Geometry: see drawing. Coordinates: mm, zero at the bounding-box minimum. A direction names the side the tool comes from. Give positions to 0.01 mm unless a question says otherwise; leave off trailing zeros. Write each loop counter-clockwise with the first axis right and the second up, starting at its lowest first coordinate (ties: lowest second). Pieces come first, ordered by that corner, then holes.
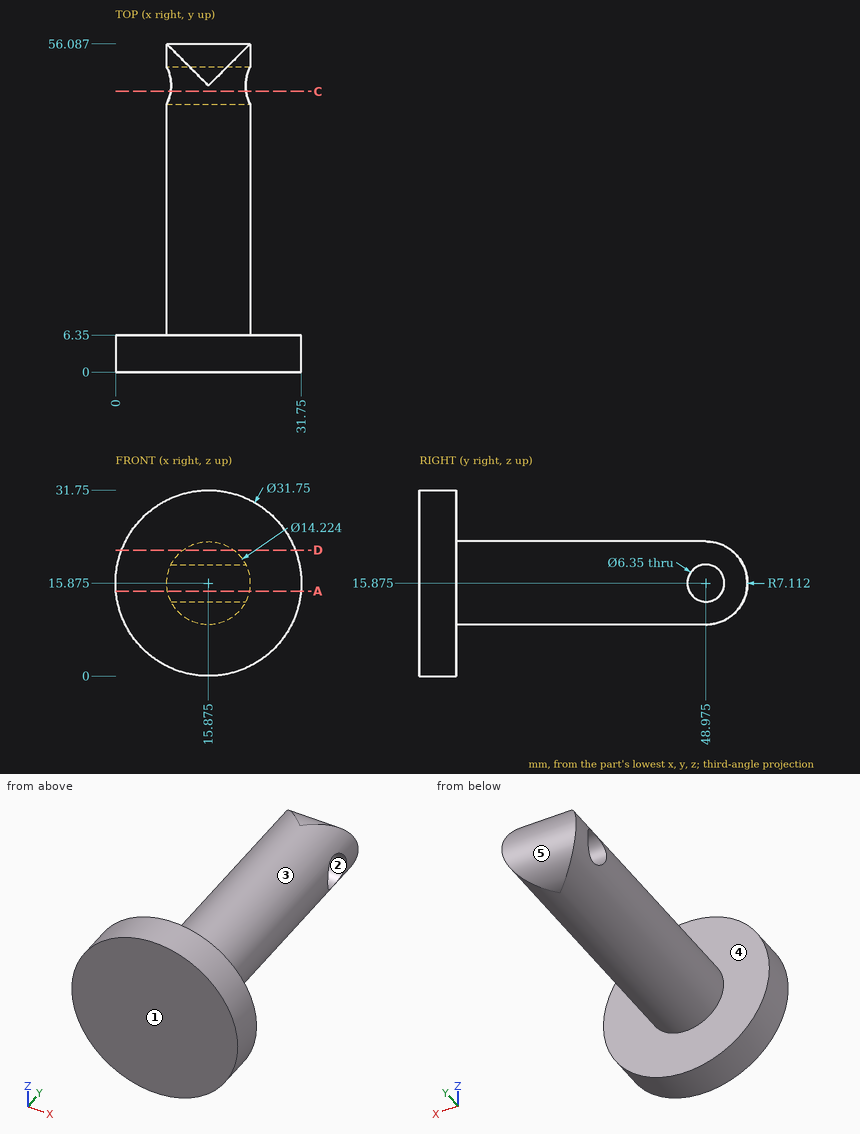
Q1. Access query for the marked faces 4 and 5. Directions: +Z, -Z, +X, -X, +Y, -Y. A direction counts if a zero-diameter tool reaches every point of the face in a straight line with its end or side. Return the directions, or none.
Q2. Section D-D, the plane z = 21.5. Return the cut outline in (x, y), then the cut area to 3 significant figures.
Q3. Material intervals for line 1 along Y through (x, z) = (22.5, 16); line 2 along Y through (x, z) = (9, 9); line 3 along Z through (x, y) = (12, 48), sorted ascending.
Q4. Section C-C, the plane y = 48. Return the cut outline in (x, z) (1 decimal).
Q5. Pin query (flat end, axial travel): pin 1 (6 mm diameter, centred on x = 22, z = 10.5, fed in from +Y); pin 2 (12 mm diameter, centred on x = 10.5, y = 40.5, fed in from +Z); pin 3 (2 mm diameter, centred on x = 22, z = 10, fed in from +Y); pin 4 (4 mm diameter, centred on y = 48.97, z = 15.88, fed in from +X). Return the tip coordinate at first contact, or that it passes through.
Q6. Mould query, pull axis Z, two halves, no side actions, for the marked faces 1, 2 and 3. Classes: +Z half, -Z half, draft (parallel to the pull), parting line (faces both ways), or undercut.
Q7. Section A-A, the plane z = 14.5. Return the cut outline in (x, y), then the cut area to 3 significant figures.
Solutions:
1. face 4: +Y
1. face 5: +X, -X, +Y
2. outline: (1.03, 0) - (30.72, 0) - (30.72, 6.35) - (20.23, 6.35) - (20.23, 53.33) - (11.52, 53.33) - (11.52, 6.35) - (1.03, 6.35) - close
2. area: 597 mm2
3. line 1: y = 0 to 45.8, 52.15 to 56.09
3. line 2: y = 0 to 6.35
3. line 3: z = 9.91 to 12.85, 18.9 to 21.84
4. outline: (9.4, 12.9) arc R7.1 ccw to (22.3, 12.9) - close; (9.4, 18.9) - (22.3, 18.9) arc R7.1 ccw to start
5. pin 1: stops at y = 55.68
5. pin 2: stops at z = 22.99
5. pin 3: stops at y = 6.35
5. pin 4: passes through
6. face 1: draft
6. face 2: undercut
6. face 3: parting line
7. outline: (0.06, 0) - (31.69, 0) - (31.69, 6.35) - (22.85, 6.35) - (22.85, 46.11) - (8.9, 46.11) - (8.9, 6.35) - (0.06, 6.35) - close; (8.9, 51.84) - (22.85, 51.84) - (22.85, 55.95) - (8.9, 55.95) - close
7. area: 813 mm2
